```python
from build123d import *

# Parameters (mm, degrees)
F1_DEPTH     = 89.69375
F2_DEPTH     = 12.7
F4_DEPTH     = 44.451
F5_T         = 2.54
F6_R         = 1.27
F7_W         = 2.54
F7_H         = 3.81
F7_H_2       = 5.08
F8_W         = 2.54
F8_H         = 3.81
F8_H_2       = 5.08
F9_DEPTH     = 12.7
F11_W        = 2.54
F11_H        = 5.08
F10_W        = 2.54
F10_H        = 5.08
F12_DEPTH    = 2.54
F13_T1_DEPTH = 18.415
F13_T3_DEPTH = 18.415


# Not quite as in the source:
# - a fillet or chamfer that OpenCascade refuses, or shapes differently, is made with other operations: its cross-section is extruded or revolved along the edge and cut away or added
# - a shell that OpenCascade refuses in one call is made with other operations: the cavity is built on its own and cut out
# - a feature names something its author has since deleted; it is built from what else it names


with BuildPart() as f1:
    # F0 (on Right) → F1 (new body, symmetric)
    with BuildSketch(Plane.YZ):
        Polygon((0, 44.45), (0, 0), (56.893405551, 44.45), align=None)
    extrude(amount=F1_DEPTH, both=True)

    # F2 (add): a face of the model
    f2_faces = [f1.faces().sort_by_distance(p)[0] for p in [
        (0, 0, 22.225),
    ]]
    extrude(f2_faces, amount=F2_DEPTH)

    # F3 (on face) → F4 (cut, through all)
    with BuildSketch(Plane.XY.offset(44.45)):
        with BuildLine():
            Line((-87.15375, -10.16), (-87.15375, -12.7))
            Line((-87.15375, -12.7), (87.15375, -12.7))
            Line((87.15375, -12.7), (87.15375, -10.16))
            ThreePointArc((87.15375, -10.16), (0, 0.1903063345), (-87.15375, -10.16))
        make_face()
    extrude(amount=-F4_DEPTH, mode=Mode.SUBTRACT)

    # F5: shell of thickness 2.54, made by hand


with BuildPart() as f5_core1:
    # F5_t2: copy of F1
    add(f1.part)

    # the walls: a layer under each face that stays
    f5_faces = [f5_core1.faces().sort_by_distance(p)[0] for p in [
        (0, 28.4467027755, 22.225),
        (89.69375, 22.0967027755, 22.225),
        (88.42375, -12.7, 22.225),
        (87.15375, -11.43, 22.225),
        (-87.15375, -11.43, 22.225),
        (-88.42375, -12.7, 22.225),
        (-89.69375, 22.0967027755, 22.225),
        (-76.7280098971, -6.35, 0),
        (50.7965296912, -2.1166666667, 0),
    ]]
    thicken(f5_faces, amount=-F5_T, mode=Mode.SUBTRACT)


with BuildPart() as f1_1:
    add(f1.part)

    # what is left inside the walls is the cavity
    f5_cavity = [f5_core1.part.solids().sort_by_distance(p)[0] for p in [
        (-29.05125, 25.930947, 23.515015),
    ]]
    add(f5_cavity, mode=Mode.SUBTRACT)

    # F6
    f6_edges = [f1_1.edges().sort_by_distance(p)[0] for p in [
        (0, 56.893406, 44.45),
    ]]
    fillet(f6_edges, radius=F6_R)

    # F7 (on face) + F8 (on face) → F9 (join)
    with BuildSketch(Plane.XZ.offset(12.7)):
        with Locations((-88.42375, 42.545)):
            Rectangle(F7_W, F7_H)
        with Locations((-88.42375, 2.54)):
            Rectangle(F7_W, F7_H_2)
    with BuildSketch(Plane.XZ.offset(12.7)):
        with Locations((88.42375, 42.545)):
            Rectangle(F8_W, F8_H)
        with Locations((88.42375, 2.54)):
            Rectangle(F8_W, F8_H_2)
    extrude(amount=F9_DEPTH)

    # F11 (on face) + F10 (on face) → F12 (join)
    with BuildSketch(Plane(origin=(0, 0, 40.64), x_dir=(1, 0, 0), z_dir=(0, 0, -1))):
        with Locations((-88.42375, 22.86)):
            Rectangle(F11_W, F11_H)
    with BuildSketch(Plane(origin=(0, 0, 40.64), x_dir=(1, 0, 0), z_dir=(0, 0, -1))):
        with Locations((88.42375, 22.86)):
            Rectangle(F10_W, F10_H)
    extrude(amount=F12_DEPTH)

    # F13: fillet of radius 3.175 on 8 edges, made by hand

    # F13_s2 → F13_t1 (cut)
    with BuildSketch(Plane.YZ.offset(79.21625)):
        with BuildLine():
            ThreePointArc((-22.225, 44.45), (-24.4700640303, 43.5200640303), (-25.4, 41.275))
            Line((-25.4, 41.275), (-25.4, 44.45))
            Line((-25.4, 44.45), (-22.225, 44.45))
        make_face()
        with BuildLine():
            ThreePointArc((-22.225, 38.1), (-24.4700640303, 39.0299359697), (-25.4, 41.275))
            Line((-25.4, 41.275), (-25.4, 38.1))
            Line((-25.4, 38.1), (-22.225, 38.1))
        make_face()
        with BuildLine():
            ThreePointArc((-25.4, 1.905), (-24.4700640303, 4.1500640303), (-22.225, 5.08))
            Line((-22.225, 5.08), (-25.4, 5.08))
            Line((-25.4, 5.08), (-25.4, 1.905))
        make_face()
        with BuildLine():
            ThreePointArc((-22.225, 0), (-24.4700640303, 0.9299359697), (-25.4, 3.175))
            Line((-25.4, 3.175), (-25.4, 0))
            Line((-25.4, 0), (-22.225, 0))
        make_face()
    extrude(amount=F13_T1_DEPTH, mode=Mode.SUBTRACT)

    # F13_s4 → F13_t3 (cut)
    with BuildSketch(Plane.YZ.offset(-97.63125)):
        with BuildLine():
            ThreePointArc((-22.225, 44.45), (-24.4700640303, 43.5200640303), (-25.4, 41.275))
            Line((-25.4, 41.275), (-25.4, 44.45))
            Line((-25.4, 44.45), (-22.225, 44.45))
        make_face()
        with BuildLine():
            ThreePointArc((-22.225, 38.1), (-24.4700640303, 39.0299359697), (-25.4, 41.275))
            Line((-25.4, 41.275), (-25.4, 38.1))
            Line((-25.4, 38.1), (-22.225, 38.1))
        make_face()
        with BuildLine():
            ThreePointArc((-25.4, 1.905), (-24.4700640303, 4.1500640303), (-22.225, 5.08))
            Line((-22.225, 5.08), (-25.4, 5.08))
            Line((-25.4, 5.08), (-25.4, 1.905))
        make_face()
        with BuildLine():
            ThreePointArc((-22.225, 0), (-24.4700640303, 0.9299359697), (-25.4, 3.175))
            Line((-25.4, 3.175), (-25.4, 0))
            Line((-25.4, 0), (-22.225, 0))
        make_face()
    extrude(amount=F13_T3_DEPTH, mode=Mode.SUBTRACT)


solid = f1_1.part
```
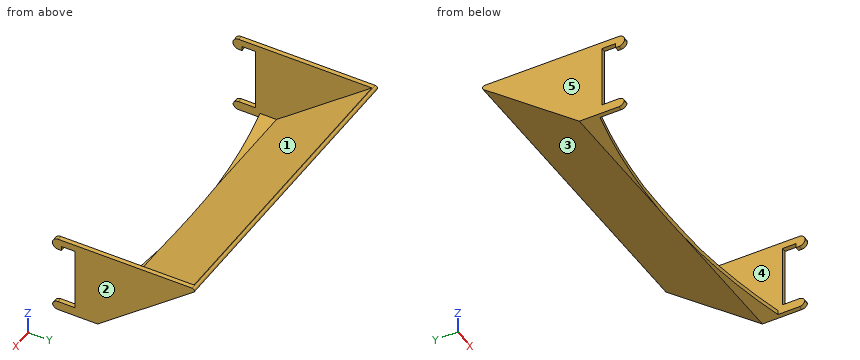
Input: part model. Units: mm. Frame: model coordinates. Face numbers are marked on the shaded views. A direction names the side the tool comes from. Give positions to 0.01 mm unless a question says otherwise; leave off trailing zeros. Order: outer loops, then holes, each group sorted by start corner. A loop starts at its lowest first (then second) coordinate and runs counter-clockwise, first axis right, second up.
1. Cut plane D-D (x = 60.5). Return loops of the section in (y, z).
Computed:
outline: (-4.76, 0) - (0, 0) - (53.99, 42.18) arc R1.27 ccw to (53.21, 44.45) - (52.77, 44.45) - (-0.87, 2.54) - (-4.76, 2.54) - close
2. Cut plane C-C (y = 10.5). Return loops of the section in (x, z), and give its area (3 significant figures).
Computed:
outline: (-89.69, 8.2) - (89.69, 8.2) - (89.69, 44.45) - (87.15, 44.45) - (87.15, 11.43) - (-87.15, 11.43) - (-87.15, 44.45) - (-89.69, 44.45) - close
area: 746 mm2
3. Pin query (flat end, axial travel): pin 1 Ø1 at (x, y) = (-51, 36.5) entering from -Z; pin 2 Ø10 at (x, z) = (19, 8.5) entering from -Y; pin 3 Ø12 at (x, y) = (-4.5, 42.5) entering from +Z; pin 4 Ø12 at (x, y) = (10, -7) entering from -Z. Return the tip coordinate at first contact, or that it passes through.
Computed:
pin 1: stops at z = 28.13
pin 2: stops at y = 0.35
pin 3: stops at z = 41.12
pin 4: passes through
4. Cut plane B-B (z = 8). Return loops of the section in (x, y).
Computed:
outline: (-89.69, -12.7) - (-87.15, -12.7) - (-87.15, 6.11) - (87.15, 6.11) - (87.15, -12.7) - (89.69, -12.7) - (89.69, 10.24) - (-89.69, 10.24) - close
5. Cut plane A-A (x = -39). Return loops of the section in (y, z).
Computed:
outline: (-1.86, 0) - (0, 0) - (53.99, 42.18) arc R1.27 ccw to (53.21, 44.45) - (52.77, 44.45) - (-0.87, 2.54) - (-1.86, 2.54) - close
6. Draft query along X for the marked faces 3, 4 and 5. Return one class per face: released by +X, released by -X, zero draft, split by the parting line, or undercut.
Computed:
face 3: zero draft
face 4: undercut
face 5: released by -X
7. Set-up query: the marked faces 1 and 2. Return all of +Z, -Z, +X, -X, +Y, -Y with unobstructed straight access to the full face (end or side cutting, diameter ignored); none if empty.
Computed:
face 1: +Z, -Y
face 2: +Z, -Z, +X, +Y, -Y
8. Line query: probe 1 along X at (y, z) = (38, 41); probe 2 along Y at (x, z) = (-37.5, 7.5); probe 3 along Z at (x, y) = (71.5, 24). Output: solid intervals per line, ascending.
Computed:
probe 1: x = -89.69 to -87.15, 87.15 to 89.69
probe 2: y = 5.47 to 9.6
probe 3: z = 18.75 to 21.97
